Input: dimensioned drawing with shaded views. Units: mm. Origin: part minimum x, y, z. A direction names the side the tool comes from. Give positions to 0.01 mm unless a question says otherwise; leave off trailing zeros. Write each loop counter-clockwise with the first axis right and the second up, starting at its lowest first coordinate (ties: lowest second). Pieces come first, ordered by that corner, then holes.
Q1. Section A-A (x = 25.4). Return the cut outline in (y, z) (1 decimal), plus the area to 3 significant figures.
Q2. Section B-B (z = 17.78). Return the cut outline in (x, y) (1 decimal).
Q3. Section D-D (x = 3.4). Return the cut outline in (y, z) (1 decimal).
Q4. Reachability of the marked faces 1 and 2 from +Z, -Z, +X, -X, +Y, -Y: full face, straight path, thin tool, end or side. Return the list, or none.
Q5. Pin query (flat end, axial travel): pin 1 Ø8.5 at (x, z) = (25.4, 71.12) entering from -Y; pin 2 Ø1.5 at (x, y) = (6, 22) entering from +Z (3 decimals); pin 3 Ø3 at (x, y) = (47.4, 25.4) entering from -Z; pin 4 Ø1 at (x, y) = (10.5, 9.5) entering from -Z. Return the tip coordinate at first contact, or that it passes through.
Q6. Section C-C (y = 47.4). Return the cut outline in (x, z) (1 decimal).
Q7. Line query: line 1 (Y direction, x = 25.4, z = 1.35); line 2 (X direction, y = 25, z = 1); line 3 (Y direction, x = 40.5, z = 47). Output: solid intervals per line, ascending.
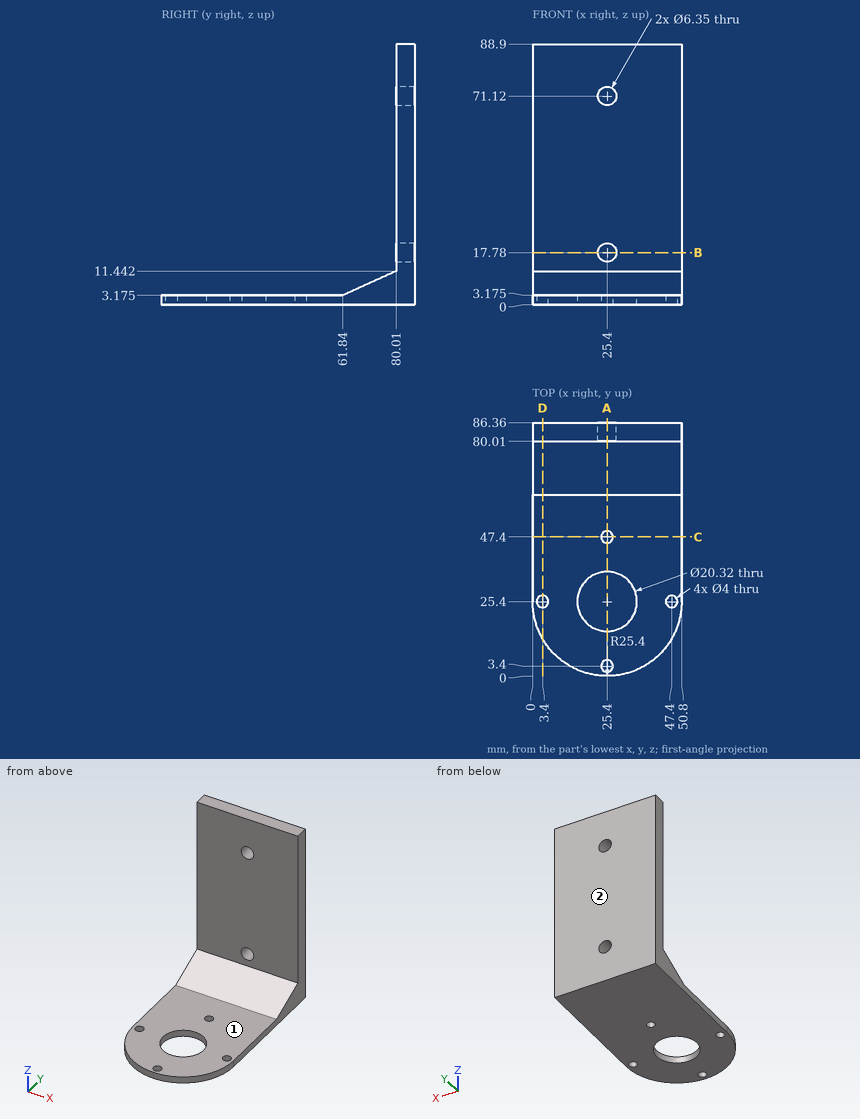
Computed:
1. outline: (0, 0) - (1.4, 0) - (1.4, 3.2) - (0, 3.2) - close; (5.4, 0) - (15.2, 0) - (15.2, 3.2) - (5.4, 3.2) - close; (35.6, 0) - (45.4, 0) - (45.4, 3.2) - (35.6, 3.2) - close; (49.4, 0) - (86.4, 0) - (86.4, 14.6) - (80, 14.6) - (80, 11.4) - (61.8, 3.2) - (49.4, 3.2) - close; (80, 21) - (86.4, 21) - (86.4, 67.9) - (80, 67.9) - close; (80, 74.3) - (86.4, 74.3) - (86.4, 88.9) - (80, 88.9) - close
1. area: 723 mm2
2. outline: (0, 80) - (22.2, 80) - (22.2, 86.4) - (0, 86.4) - close; (28.6, 80) - (50.8, 80) - (50.8, 86.4) - (28.6, 86.4) - close
3. outline: (12.7, 0) - (23.4, 0) - (23.4, 3.2) - (12.7, 3.2) - close; (27.4, 0) - (86.4, 0) - (86.4, 88.9) - (80, 88.9) - (80, 11.4) - (61.8, 3.2) - (27.4, 3.2) - close
4. face 1: +Z, +X, -X, -Y
4. face 2: +Z, -Z, +X, -X, +Y
5. pin 1: stops at y = 80.01
5. pin 2: stops at z = 3.175
5. pin 3: passes through
5. pin 4: stops at z = 0
6. outline: (0, 0) - (23.4, 0) - (23.4, 3.2) - (0, 3.2) - close; (27.4, 0) - (50.8, 0) - (50.8, 3.2) - (27.4, 3.2) - close
7. line 1: y = 0 to 1.4, 5.4 to 15.24, 35.56 to 45.4, 49.4 to 86.36
7. line 2: x = 0 to 1.44, 5.36 to 15.25, 35.55 to 45.44, 49.36 to 50.8
7. line 3: y = 80.01 to 86.36
